from build123d import *

# Parameters (mm, degrees)
SKETCH_1_W          = 68
SKETCH_1_H          = 50
SKETCH_1_R          = 3
EXTRUDE_1_DEPTH     = 6
SKETCH_3_W          = 68
SKETCH_3_H          = 6
EXTRUDE_2_DEPTH     = 50
CUT_EXTRUDE_1_REACH = 8
SKETCH_4_R          = 13
SKETCH_4_R_2        = 3.5


with BuildPart() as part:
    # 草图1 → 凸台-拉伸1 (new body)
    with BuildSketch(Plane(origin=(0, 0, 0), x_dir=(1, 0, 0), z_dir=(0, 1, 0))):
        with Locations((0, 25)):
            Rectangle(SKETCH_1_W, SKETCH_1_H)
        with Locations((-27.5, 35)):
            Circle(SKETCH_1_R, mode=Mode.SUBTRACT)
        with Locations((27.5, 35)):
            Circle(SKETCH_1_R, mode=Mode.SUBTRACT)
        with Locations((-27.5, 15)):
            Circle(SKETCH_1_R, mode=Mode.SUBTRACT)
        with Locations((27.5, 15)):
            Circle(SKETCH_1_R, mode=Mode.SUBTRACT)
    extrude(amount=EXTRUDE_1_DEPTH)

    # 草图3 → 凸台-拉伸2 (add)
    with BuildSketch(Plane(origin=(0, 6, 0), x_dir=(1, 0, 0), z_dir=(0, 1, 0))):
        with Locations((0, 47)):
            Rectangle(SKETCH_3_W, SKETCH_3_H)
    extrude(amount=-EXTRUDE_2_DEPTH)

    # 草图4 → 切除-拉伸1 (cut, up to next)
    with BuildSketch(Plane.XY.offset(-44), mode=Mode.PRIVATE) as cut_extrude_1_sk1:
        with Locations((0, -18)):
            Circle(SKETCH_4_R)
    cut_extrude_1_tool1 = extrude(cut_extrude_1_sk1.sketch, amount=-CUT_EXTRUDE_1_REACH, mode=Mode.PRIVATE) & part.part
    add(cut_extrude_1_tool1.solids().sort_by_distance((0, -18, -44))[0], mode=Mode.SUBTRACT)
    # 草图4 → 切除-拉伸1 (cut, up to next)
    with BuildSketch(Plane.XY.offset(-44), mode=Mode.PRIVATE) as cut_extrude_1_sk2:
        with Locations((28, -18)):
            Circle(SKETCH_4_R_2)
    cut_extrude_1_tool2 = extrude(cut_extrude_1_sk2.sketch, amount=-CUT_EXTRUDE_1_REACH, mode=Mode.PRIVATE) & part.part
    add(cut_extrude_1_tool2.solids().sort_by_distance((28, -18, -44))[0], mode=Mode.SUBTRACT)
    # 草图4 → 切除-拉伸1 (cut, up to next)
    with BuildSketch(Plane.XY.offset(-44), mode=Mode.PRIVATE) as cut_extrude_1_sk3:
        with Locations((-28, -18)):
            Circle(SKETCH_4_R_2)
    cut_extrude_1_tool3 = extrude(cut_extrude_1_sk3.sketch, amount=-CUT_EXTRUDE_1_REACH, mode=Mode.PRIVATE) & part.part
    add(cut_extrude_1_tool3.solids().sort_by_distance((-28, -18, -44))[0], mode=Mode.SUBTRACT)


solid = part.part
Design review of the part built by this model. Coordinates are the model's own, in mm. A direction names the side the tool comes from. Give positions to 0.01 mm unless a question says otherwise; leave off trailing zeros. Loops run counter-clockwise (first coordinate to the right, second up) from the corner with the lowest first, then second, coordinate; pieces in that order, holes last. Notation, with made-up numbers: (-39.5, 55) - (13.5, 55) arc R19 cw to (13.5, 83) - close; hole circle Ø5 at (61.25, 27). An arc over 180 degrees is marked (long way). Use CSV: the item, a comma, the result in double quotes. Start each with the question number.
1. Draft analysis for pull direction Z (two halves, no side actions). For faces 3 (the cylindrical face through (29.88, -15.05, -46.96)), 4 (the cylindrical face through (-29.71, 2.96, -37.03)), 5 (the flat face through (7, -30, -50)), 6 (the cylindrical face through (25.1, 3, -13.2)), state which applies: released by +Z, released by -Z, zero draft, split by the parting line, or undercut.
2. Wall thickness on L1, parallel to X at y = 4.5, z = -35; L2, parallel to Z at x = 27.5, y = 2.3; L3, parallel to Y at x = 28, z = -46: over which ranges is each line inside the solid? List them lowest first.
3. Add section C-C (y = -26.5). State the section outline as (x, z) points, plus the area to 3 significant figures.
4. Add section A-A (y = -18). State the section outline as (x, z) points.
5. Machinability: for faces 1 (the flat face through (-0.5, -31.5, -44)), 2 (the flat face through (0, -44, -47)), which of the approach directions +Z, -Z, +X, -X, +Y, -Y give a long, thin tool a straight path to every point of the face, cutting with its end or side? Answer none if there is none.
6. Add section D-D (z = -17). State the section outline as (x, y) points.
7. Insertion check: P1, Ø7, axis at x = 27.5, z = -15, coming from the -Y side; P2, Ø8, axis at x = 27.5, z = -35, coming from the +Y side; P3, Ø1.5, axis at x = -20.5, y = -8.5, coming from the +Z side. Each pin has a flat end and moves straight along its axis. Give the tip position at first contact, or say it passes through.
8. Add section B-B (x = -5). State the section outline as (y, z) points.
Results found:
1,face 3,"zero draft"
1,face 4,"undercut"
1,face 5,"released by -Z"
1,face 6,"undercut"
2,L1,"x = -34 to -30.5, -24.5 to 24.5, 30.5 to 34"
2,L2,"z = -50 to -38, -32 to -18, -12 to 0"
2,L3,"y = -44 to -21.5, -14.5 to 6"
3,outline,"(-34, -50) - (-9.84, -50) - (-9.84, -44) - (-34, -44) - close; (9.84, -50) - (34, -50) - (34, -44) - (9.84, -44) - close"
3,area,"290 mm²"
4,outline,"(-34, -50) - (-31.5, -50) - (-31.5, -44) - (-34, -44) - close; (-24.5, -50) - (-13, -50) - (-13, -44) - (-24.5, -44) - close; (13, -50) - (24.5, -50) - (24.5, -44) - (13, -44) - close; (31.5, -50) - (34, -50) - (34, -44) - (31.5, -44) - close"
5,face 1,"+Z, +X, -X, -Y"
5,face 2,"+Z, -Z, +X, -X, -Y"
6,outline,"(-34, 0) - (-29.74, 0) - (-29.74, 6) - (-34, 6) - close; (-25.26, 0) - (25.26, 0) - (25.26, 6) - (-25.26, 6) - close; (29.74, 0) - (34, 0) - (34, 6) - (29.74, 6) - close"
7,P1,"stops at y = 0"
7,P2,"stops at y = 6"
7,P3,"stops at z = -44"
8,outline,"(-44, -50) - (-30, -50) - (-30, -44) - (-44, -44) - close; (-6, -50) - (6, -50) - (6, 0) - (0, 0) - (0, -44) - (-6, -44) - close"
